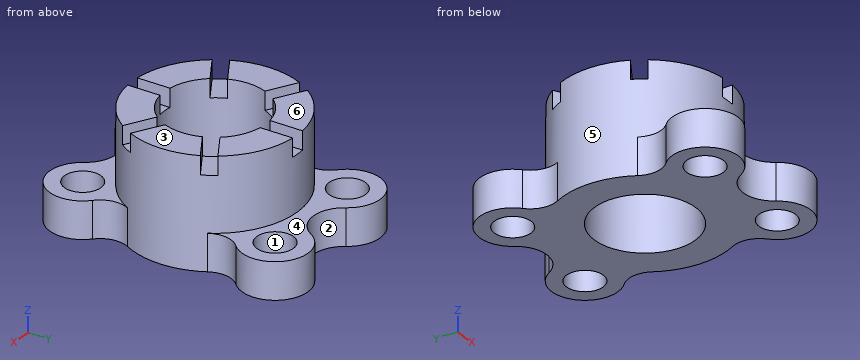
Autodesk Fusion 360 part; units mm, degrees
sketch "Sketch1" plane through (0, 0, 0) normal (0, 0, 1) x (1, 0, 0)
  circle A0 centre (0, 0) radius 275
  circle A1 centre (0, 0) radius 450
  line L0 (0, 0) -> (0, 1300) construction
  line L1 (0, 0) -> (1400, 0) construction
  line L2 (0, 0) -> (-820.061, 1420.3873) construction
  circle A2 centre (-300, 519.6152) radius 100
  circle A3 centre (300, 519.6152) radius 100
  arc A4 (-145.7143, 612.3294) -> (145.7143, 612.3294) centre (0, 699.8928) ccw
  arc A5 (-394.2776, 216.899) -> (-422.0297, 387.2946) centre (-516.9418, 284.3786) ccw
  arc A6 (422.0297, 387.2946) -> (394.2776, 216.899) centre (516.9418, 284.3786) ccw
  arc A7 (-145.7143, 612.3294) -> (-422.0297, 387.2946) centre (-300, 519.6152) ccw
  arc A8 (422.0297, 387.2946) -> (145.7143, 612.3294) centre (300, 519.6152) ccw
  arc A9 (-422.0297, -387.2946) -> (-394.2776, -216.899) centre (-516.9418, -284.3786) ccw
  arc A10 (-422.0297, -387.2946) -> (-145.7143, -612.3294) centre (-300, -519.6152) ccw
  arc A11 (145.7143, -612.3294) -> (-145.7143, -612.3294) centre (0, -699.8928) ccw
  arc A12 (145.7143, -612.3294) -> (422.0297, -387.2946) centre (300, -519.6152) ccw
  arc A13 (394.2776, -216.899) -> (422.0297, -387.2946) centre (516.9418, -284.3786) ccw
  circle A14 centre (-300, -519.6152) radius 100
  circle A15 centre (300, -519.6152) radius 100
  dimension "d1" = 550
  dimension "d2" = 900
  dimension "d3" = 30
  dimension "d4" = 200
  dimension "d5" = 360
  dimension "d6" = 600
  dimension "d7" = 170
  dimension "d8" = 140
extrude "Extrude1" add sketch "Sketch1" along normal blind 200 contours A1 A4 A5 A6 A7 A8 | A1 A9 A10 A11 A12 A13 makes body 1 at (-383.5434, 235.3603, 133.3333) makes body 2 at (383.5434, -235.3603, 133.3333)
extrude "Extrude2" add sketch "Sketch1" along normal blind 600 contours A1 bodies 1 2
sketch "Sketch2" plane through (0, 0, 600) normal (0, 0, 1) x (-1, 0, 0)
  circle A0 centre (0, 0) radius 275
  circle A1 centre (0, 0) radius 450
  line L0 (37.0395, -264.2232) -> (-42.9605, -264.2232)
  line L1 (-42.9605, -264.2232) -> (-42.9605, -454.2232)
  line L2 (-42.9605, -454.2232) -> (37.0395, -454.2232)
  line L3 (37.0395, -454.2232) -> (37.0395, -264.2232)
  line L4 (37.0395, -264.2232) -> (-42.9605, -454.2232) construction
  line L5 (-42.9605, -264.2232) -> (37.0395, -454.2232) construction
  point P0 (-2.9605, -359.2232)
  dimension "d13" = 80
  dimension "d14" = 190
extrude "Extrude3" cut sketch "Sketch2" against normal blind 100 contours A0 A1 L1 L3 picked at (28.1553, -331.9237) bodies 1
pattern_circular "C-Pattern1" count 6 over 360 about axis through (0, 0, 600) along (0, 0, 1) of "Extrude3"
The model under review builds one solid part; all positions refer to its coordinate system, in mm. Face numbers are marked on the shaded views. A direction names the side the tool comes from. Round coordinates to 2 decimals unless told otherwise and drop trailing zeros. Loops run counter-clockwise (first coordinate to the right, second up) from the corner with the lowest first, then second, coordinate; pieces in that order, holes last. Notation, with made-up numbers: (51.5, 22.5) -> (55.5, 22.5) arc R5 ccw to (55.5, 31.5) -> close; hole circle Ø7 at (-2.5, -29). An arc over 180 degrees is marked (long way). One line per question, with ' | ' between items. Start each with the question number.
Item 1: For pin 1 (3 mm diameter, centred on y = -147.5, z = 423.5, fed in from -X); pin 2 (4 mm diameter, centred on y = 100, z = 514, fed in from +X); pin 3 (4 mm diameter, centred on x = 251, z = 220, fed in from +Y), all flat-tipped, find the tip position at first contact; note any pin that passes through.
Item 2: Draft analysis for pull direction Y (two halves, no side actions). For the marked faces 1, 2 and 3, state which applies: +Y half, -Y half, draft (parallel to the pull), parting line (faces both ways), or undercut.
Item 3: Add section B-B, the plane x = 0. Write out the cut boundary in (y, z), then the cut area to 3 significant figures.
Item 4: Machinability: for the marked faces 4, 5 and 6, which of the approach directions +Z, -Z, +X, -X, +Y, -Y give a long, thin tool a straight path to every point of the face, cutting with its end or side? Answer none if there is none.
Item 5: Wall thickness on line 1 along Y through (x, z) = (300, 72.5); line 2 along Y through (x, z) = (-338, 46); line 3 along X through (y, z) = (-570.5, 81): over which ranges is each line inside the solid? List them lowest first. Write a range as [from, to].
Item 6: Add section A-A, the plane y = 0. Write out the cut boundary in (x, z).
Item 7: Add section C-C, the plane x = 300. Write out the cut boundary in (y, z), then the cut area to 3 significant figures.
Item 8: Add section D-D, the plane z = 389. Write out the cut boundary in (x, y).
Return value:
1) pin 1: stops at x = -425.66 | pin 2: stops at x = 439.2 | pin 3: stops at y = 374.83
2) face 1: undercut | face 2: +Y half | face 3: draft
3) outline: (-529.89, 0) -> (-275, 0) -> (-275, 500) -> (-450, 500) -> (-450, 200) -> (-529.89, 200) -> close; (275, 0) -> (529.89, 0) -> (529.89, 200) -> (450, 200) -> (450, 500) -> (275, 500) -> close | area: 207,000 mm2
4) face 4: +Z, +Y | face 5: +Z | face 6: +Z, +X, -X, +Y, -Y
5) line 1: y = [-699.62, -619.62], [-419.62, 419.62], [619.62, 699.62] | line 2: y = [-695.56, -612.11], [-427.12, 427.12], [612.11, 695.56] | line 3: x = [-472.66, -386.09], [-213.91, -110.26], [110.26, 213.91], [386.09, 472.66]
6) outline: (-450, 0) -> (-275, 0) -> (-275, 600) -> (-450, 600) -> close; (275, 0) -> (450, 0) -> (450, 600) -> (275, 600) -> close
7) outline: (-699.62, 0) -> (-619.62, 0) -> (-619.62, 200) -> (-699.62, 200) -> close; (-419.62, 0) -> (419.62, 0) -> (419.62, 200) -> (335.41, 200) -> (335.41, 600) -> (215.97, 600) -> (215.97, 500) -> (123.6, 500) -> (123.6, 600) -> (-130.44, 600) -> (-130.44, 500) -> (-222.81, 500) -> (-222.81, 600) -> (-335.41, 600) -> (-335.41, 200) -> (-419.62, 200) -> close; (619.62, 0) -> (699.62, 0) -> (699.62, 200) -> (619.62, 200) -> close | area: 450,000 mm2
8) outline: circle Ø900 at (0, 0); hole circle Ø550 at (0, 0)
